Design review of the part built by this model. Coordinates are the model's own, in mm. Face numbers are marked on the shaded views. A direction names the side the tool comes from. Coordinates: 2 decimals unless noted, no trailing zeros. Write each loop counter-clockwise with the first axis right and the second up, starting at its lowest first coordinate (ties: lowest second). Pieces come first, ordered by that corner, then holes. Notation, with made-up numbers: (69.25, -21.5) - (106.25, -21.5) arc R6 cw to (106.25, -10.5) - close; hole circle Ø1 at (86, 4.5). An arc over 180 degrees is marked (long way). One line per item, written item: value.
from build123d import *

# Parameters (mm, degrees)
SKETCH_1_R      = 1.6
EXTRUDE_1_DEPTH = 3
FILLET_1_R      = 0.5
FILLET_2_R      = 2
EXTRUDE_2_DEPTH = 3
FILLET_3_R      = 1


with BuildPart() as part:
    # ｽｹｯﾁ1 → ﾎﾞｽ - 押し出し1 (new body)
    with BuildSketch(Plane.XY):
        Polygon((0, -19), (0, 19), (17, 19), (17, 11.3), (5.5, 11.3), (5.5, -11.3), (17, -11.3), (17, -19), align=None)
        with Locations((11.5, 14)):
            Circle(SKETCH_1_R, mode=Mode.SUBTRACT)
        with Locations((11.5, -14)):
            Circle(SKETCH_1_R, mode=Mode.SUBTRACT)
    extrude(amount=EXTRUDE_1_DEPTH)

    # ﾌｨﾚｯﾄ1
    fillet_1_edges = [part.edges().sort_by_distance(p)[0] for p in [
        (5.5, 11.3, 1.5),
        (5.5, -11.3, 1.5),
    ]]
    fillet(fillet_1_edges, radius=FILLET_1_R)

    # ﾌｨﾚｯﾄ2
    fillet_2_edges = [part.edges().sort_by_distance(p)[0] for p in [
        (17, 19, 1.5),
        (17, -19, 1.5),
    ]]
    fillet(fillet_2_edges, radius=FILLET_2_R)

    # ｽｹｯﾁ2 → ﾎﾞｽ - 押し出し2 (add)
    with BuildSketch(Plane.XY.offset(3)):
        Polygon((5.5, 19), (5.5, 24), (15, 19), align=None)
        Polygon((5.5, -19), (5.5, -24), (15, -19), align=None)
    extrude(amount=-EXTRUDE_2_DEPTH)

    # ﾌｨﾚｯﾄ3
    fillet_3_edges = [part.edges().sort_by_distance(p)[0] for p in [
        (15, 19, 1.5),
        (15, -19, 1.5),
    ]]
    fillet(fillet_3_edges, radius=FILLET_3_R)


solid = part.part
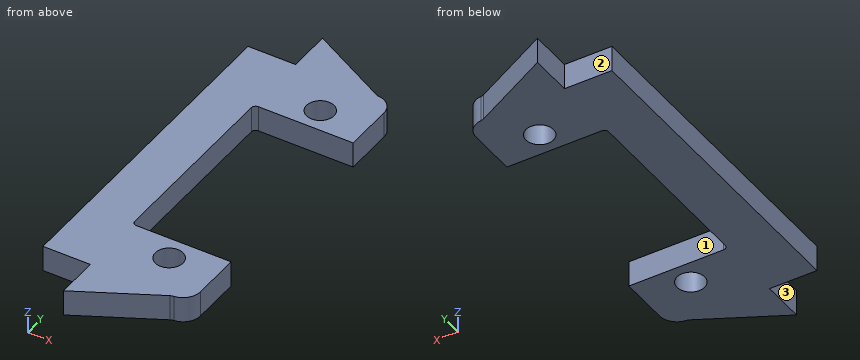
1. Consider section A-A, the plane y = 14. Write out the cut boundary in (x, z), then the cut area to 3 significant figures.
Answer block:
outline: (0, 0) - (9.9, 0) - (9.9, 3) - (0, 3) - close; (13.1, 0) - (17, 0) - (17, 3) - (13.1, 3) - close
area: 41.4 mm^2
2. Insertion check: pin 1 Ø0.9 at (x, z) = (13, 1.5) entering from +Y; pin 2 Ø1 at (x, z) = (9.5, 2) entering from -Y; pin 3 Ø1.5 at (x, z) = (3, 1) entering from +Y; pin 4 Ø2.5 at (x, y) = (11.5, 14) entering from -Z. Each pin has a flat end and moves straight along its axis. Give the tip position at first contact, or say it passes through.
Answer block:
pin 1: stops at y = 20.29
pin 2: stops at y = -22.16
pin 3: stops at y = 19
pin 4: passes through
3. For the marked faces 1, 2 and 3, list the 3-axis set-ups (+Z, -Z, +X, -X, +Y, -Y) from which the entire face can be reached by the end or side of a thin tool; tool diameter is ignored.
Answer block:
face 1: +Z, -Z, +X
face 2: +Z, -Z, -X, +Y
face 3: +Z, -Z, -X, -Y
4. Consider section D-D, the plane x = 8.25. Write out the cut boundary in (y, z), then the cut area to 3 significant figures.
Answer block:
outline: (-22.55, 0) - (-11.3, 0) - (-11.3, 3) - (-22.55, 3) - close; (11.3, 0) - (22.55, 0) - (22.55, 3) - (11.3, 3) - close
area: 67.5 mm^2
5. Consider section B-B, the plane z = 2.5. Write out the cut boundary in (x, y), then the cut area to 3 significant figures.
Answer block:
outline: (0, -19) - (5.5, -19) - (5.5, -24) - (14.8, -19.1) arc R1 cw to (15.18, -18.99) arc R2 ccw to (17, -17) - (17, -11.3) - (6, -11.3) arc R0.5 cw to (5.5, -10.8) - (5.5, 10.8) arc R0.5 cw to (6, 11.3) - (17, 11.3) - (17, 17) arc R2 ccw to (15.18, 18.99) arc R1 cw to (14.8, 19.1) - (5.5, 24) - (5.5, 19) - (0, 19) - close; hole circle Ø3.2 at (11.5, -14); hole circle Ø3.2 at (11.5, 14)
area: 416 mm^2
6. Consider section C-C, the plane x = 12.25. Write out the cut boundary in (y, z), then the cut area to 3 significant figures.
Answer block:
outline: (-20.45, 0) - (-15.41, 0) - (-15.41, 3) - (-20.45, 3) - close; (-12.59, 0) - (-11.3, 0) - (-11.3, 3) - (-12.59, 3) - close; (11.3, 0) - (12.59, 0) - (12.59, 3) - (11.3, 3) - close; (15.41, 0) - (20.45, 0) - (20.45, 3) - (15.41, 3) - close
area: 37.9 mm^2
7. Wall thickness on line 1 along Y through (x, z) = (11.5, 0.7); line 2 along Y through (x, z) = (3.75, 2.55); line 3 along X through (y, z) = (0, 2.25): over which ranges is each line inside the solid? List them lowest first.
Answer block:
line 1: y = -20.84 to -15.6, -12.4 to -11.3, 11.3 to 12.4, 15.6 to 20.84
line 2: y = -19 to 19
line 3: x = 0 to 5.5
